```python
from build123d import *

# Parameters (mm, degrees)
ESQUISSE1_W             = 22
ESQUISSE1_H             = 462
BOSS_EXTRU_1_DEPTH      = 73.5
ESQUISSE2_W             = 38.5
ESQUISSE2_H             = 25
ENL_V_MAT_EXTRU_1_DEPTH = 35
ESQUISSE3_W             = 23.5
ESQUISSE3_H             = 323
ENL_V_MAT_EXTRU_2_DEPTH = 35


with BuildPart() as part:
    # Esquisse1 → Boss.-Extru.1 (new body)
    with BuildSketch(Plane.XY):
        with Locations((129, 30)):
            Rectangle(ESQUISSE1_W, ESQUISSE1_H)
    extrude(amount=BOSS_EXTRU_1_DEPTH)

    # Esquisse2 → Enlèv. mat.-Extru.1 (cut)
    with BuildSketch(Plane.ZY.offset(-118)):
        with Locations((19.25, 0.5)):
            Rectangle(ESQUISSE2_W, ESQUISSE2_H)
    extrude(amount=-ENL_V_MAT_EXTRU_1_DEPTH, mode=Mode.SUBTRACT)

    # Esquisse3 → Enlèv. mat.-Extru.2 (cut)
    with BuildSketch(Plane(origin=(140, 0, 0), x_dir=(0, 0, -1), z_dir=(1, 0, 0))):
        with Locations((-11.75, 0.5)):
            Rectangle(ESQUISSE3_W, ESQUISSE3_H)
    extrude(amount=-ENL_V_MAT_EXTRU_2_DEPTH, mode=Mode.SUBTRACT)


solid = part.part
```
Can you work these out from the model? Positions are in its coordinate system, mm. A direction names the side the tool comes from. Round coordinates to 2 decimals unless told otherwise and drop trailing zeros. Loops run counter-clockwise (first coordinate to the right, second up) from the corner with the lowest first, then second, coordinate; pieces in that order, holes last.
Item 1: Suppose I cut it at B-B, the plane x = 131. Write out the boundary of the cut face in (y, z), then the cut area to 3 significant figures.
Item 2: Suppose I cut it at A-A, the plane z = 6. Write out the boundary of the cut face in (x, y), then the cut area to 3 significant figures.
Item 3: Will these pins go through, and if not, where does the flat tip stop? pin 1 Ø6.5 at (x, y) = (134, -83.5) entering from -Z; pin 2 Ø12 at (x, y) = (126, -3.5) entering from -Z.
Item 4: Suppose I cut it at C-C, the plane y = 8.5. Write out the boundary of the cut face in (x, z), then the cut area to 3 significant figures.
Item 5: If we mould it in two halves opening along Y, with no side actions, what happens to faces 1 (the flat face through (129, -201, 36)), 2 (the flat face through (129, 33, 73.5)), 3 (the flat face through (129, 0, 38.5))? For each: +Y half, -Y half, draft (parallel to the pull), parting line (faces both ways), or undercut.
Item 6: Which directions (+Z, -Z, +X, -X, +Y, -Y) give clear straight access to the entire face, cutting with the end or side of a thin tool? Please do faces 4 (the flat face through (129, 13, 31)), 5 (the flat face through (129, 261, 36)).
Item 7: Suppose I cut it at D-D, the plane z = 32.5. Write out the boundary of the cut face in (x, y), then the cut area to 3 significant figures.
Item 8: Please list where these lines run through material, in increasing order: L1, parallel to Y at x = 132.5, z = 19; L2, parallel to Y at x = 121.25, z = 35; L3, parallel to Z at x = 127.25, y = -113.
Reported:
1. outline: (-201, 0) - (-161, 0) - (-161, 23.5) - (-12, 23.5) - (-12, 38.5) - (13, 38.5) - (13, 23.5) - (162, 23.5) - (162, 0) - (261, 0) - (261, 73.5) - (-201, 73.5) - close
1. area: 26,000 mm2
2. outline: (118, -201) - (140, -201) - (140, -161) - (118, -161) - close; (118, 162) - (140, 162) - (140, 261) - (118, 261) - close
2. area: 3,060 mm2
3. pin 1: stops at z = 23.5
3. pin 2: stops at z = 38.5
4. outline: (118, 38.5) - (140, 38.5) - (140, 73.5) - (118, 73.5) - close
4. area: 770 mm2
5. face 1: -Y half
5. face 2: draft
5. face 3: undercut
6. face 4: -Z, +X, -X
6. face 5: +Z, -Z, +X, -X, +Y
7. outline: (118, -201) - (140, -201) - (140, -12) - (118, -12) - close; (118, 13) - (140, 13) - (140, 261) - (118, 261) - close
7. area: 9,610 mm2
8. L1: y = -201 to -161, 162 to 261
8. L2: y = -201 to -12, 13 to 261
8. L3: z = 23.5 to 73.5
